The model under review builds one solid part; all positions refer to its coordinate system, in mm. Coordinates: 2 decimals unless noted, no trailing zeros. Write each loop counter-clockwise with the first axis right and the second up, starting at its lowest first coordinate (ties: lowest second). Pieces come first, ordered by that corner, then holes. Notation, with made-up numbers: M 46,75 L 100,75 A21 cw 100,81 Z; hole C 40,44 d7. An arc over 180 degrees is marked long. Answer as a JSON object with one key per item and string values.
```python
from build123d import *

# Parameters (mm, degrees)
CHAMFER1_SIZE = 0.5


with BuildPart() as part:
    # Sketch1 → Revolve1 (revolve)
    with BuildSketch(Plane.XY):
        Polygon((3, 0), (3, 9.5), (6, 9.5), (6, 6.75), (5.75, 6.75), (5.75, 5.65), (6, 5.65), (6, 0), align=None)
    revolve(axis=Axis((0, 0, 0), (0, 1, 0)))

    # Chamfer1
    chamfer1_edges = [part.edges().sort_by_distance(p)[0] for p in [
        (-6, 9.5, 0),
    ]]
    chamfer(chamfer1_edges, length=CHAMFER1_SIZE)

    # Mirror1: part across plane


with BuildPart() as part_1:
    add(part.part)
    add(part.part.mirror(Plane(origin=(6, 0, 0), x_dir=(0, 0, 1), z_dir=(0, -1, 0))))


solid = part_1.part
```
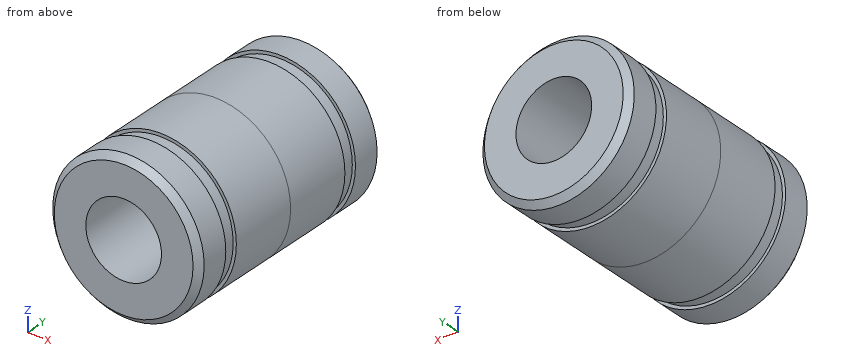
(1) Wall thickness on line 1 along X through (y, z) = (2, 0); line 2 along X through (y, z) = (-2.5, -0.75): over which ranges is each line inside the solid? List them lowest first. Write a range as from..to.
Results list:
{"line 1": "-6..-3, 3..6", "line 2": "-5.95..-2.9, 2.9..5.95"}
(2) Add section D-D on y = -7.75. Give the boundary of the cut face in (x, z), and give its area (3 significant figures).
Results list:
{"outline": "C 0,0 d12; hole C 0,0 d6", "area": "84.8 mm²"}
(3) For pin 1 Ø1 at (y, z) = (-7.5, 4.5) entering from +X; pin 2 Ø5 at (x, z) = (0, 0) entering from -Y; pin 3 Ø1 at (y, z) = (6.5, -4.5) entering from +X; pin 4 Ø3.5 at (x, z) = (2.5, -1.5) entering from -Y, all flat-tipped, find the tip position at first contact; note any pin that passes through.
Results list:
{"pin 1": "x = 4.47", "pin 2": "through", "pin 3": "x = 4.41", "pin 4": "y = -9.5"}
(4) Add section C-C on y = 6. Give the boundary of the cut face in (x, z).
Results list:
{"outline": "C 0,0 d11.5; hole C 0,0 d6"}
(5) Add section B-B on z = 0. Give the boundary of the cut face in (x, y).
Results list:
{"outline": "M -6,-9 L -5.5,-9.5 L -3,-9.5 L -3,9.5 L -5.5,9.5 L -6,9 L -6,6.75 L -5.75,6.75 L -5.75,5.65 L -6,5.65 L -6,-5.65 L -5.75,-5.65 L -5.75,-6.75 L -6,-6.75 Z; M 3,-9.5 L 5.5,-9.5 L 6,-9 L 6,-6.75 L 5.75,-6.75 L 5.75,-5.65 L 6,-5.65 L 6,5.65 L 5.75,5.65 L 5.75,6.75 L 6,6.75 L 6,9 L 5.5,9.5 L 3,9.5 Z"}
(6) Add section A-A on x = 0. Give the boundary of the cut face in (y, z).
Results list:
{"outline": "M -9.5,-5.5 L -9,-6 L -6.75,-6 L -6.75,-5.75 L -5.65,-5.75 L -5.65,-6 L 5.65,-6 L 5.65,-5.75 L 6.75,-5.75 L 6.75,-6 L 9,-6 L 9.5,-5.5 L 9.5,-3 L -9.5,-3 Z; M -9.5,3 L 9.5,3 L 9.5,5.5 L 9,6 L 6.75,6 L 6.75,5.75 L 5.65,5.75 L 5.65,6 L -5.65,6 L -5.65,5.75 L -6.75,5.75 L -6.75,6 L -9,6 L -9.5,5.5 Z"}
